```python
from build123d import *

# Parameters (mm, degrees)
F0_R     = 73.412381
F1_DEPTH = 25.4
F2_W     = 16.572997
F2_H     = 80.379516
F3_DEPTH = 25.4


with BuildPart() as f1:
    # F0 (on Top) → F1 (new body)
    with BuildSketch(Plane.XY):
        Circle(F0_R)
    extrude(amount=F1_DEPTH)

    # F2 (on face) → F3 (join)
    with BuildSketch(Plane.XY.offset(25.4)):
        with Locations((-12.828204, 0)):
            Rectangle(F2_W, F2_H)
    extrude(amount=F3_DEPTH)


solid = f1.part
```
For this review, take the finished solid that the model builds, in its own axes (mm). A direction names the side the tool comes from. Coordinates: 2 decimals unless noted, no trailing zeros. Order: outer loops, then holes, each group sorted by start corner. A loop starts at its lowest first (then second) coordinate and runs counter-clockwise, first axis right, second up. Notation, with made-up numbers: (2.25, 73.25) -> (38.25, 73.25) arc R21 ccw to (38.25, 85.25) -> close; hole circle Ø4 at (2.25, 84.25). An arc over 180 degrees is marked (long way). Answer as CSV lines item,"result".
Q1. Wall thickness on line 1 along Z through (x, y) = (4, -14); line 2 along Y through (x, z) = (-18, 40); line 3 along X through (y, z) = (11.5, 32.5): over which ranges is each line inside the solid? List them lowest first. Write a range as [from, to].
Model answer:
line 1,"z = [0, 25.4]"
line 2,"y = [-40.19, 40.19]"
line 3,"x = [-21.11, -4.54]"
Q2. We need section C-C (x = 0). State the section outline as (y, z) points, plus the area to 3 significant figures.
Model answer:
outline,"(-73.41, 0) -> (73.41, 0) -> (73.41, 25.4) -> (-73.41, 25.4) -> close"
area,"3,730 mm2"
Q3. Clearance check with flat-ended pins moving along their axes: pin 1 Ø1 at (x, z) = (-36.5, 15.5) entering from +Y; pin 2 Ø6 at (y, z) = (43, 37) entering from +X; pin 3 Ø1.5 at (x, z) = (12, 21.5) entering from +Y; pin 4 Ø6 at (x, y) = (-27.5, 47) entering from -Z. State where each tip first meets the part, or that it passes through.
Model answer:
pin 1,"stops at y = 63.98"
pin 2,"stops at x = -4.54"
pin 3,"stops at y = 72.55"
pin 4,"stops at z = 0"
Q4. For faces 1 (the face through (-13, 1, 50.8)), 2 (the face through (-21.115, -1, 38)), 3 (the face through (-4.542, -1, 38)), list the 3-axis set-ups (+Z, -Z, +X, -X, +Y, -Y) from which the entire face can be reached by the end or side of a thin tool; tool diameter is ignored.
Model answer:
face 1,"+Z, +X, -X, +Y, -Y"
face 2,"+Z, -X, +Y, -Y"
face 3,"+Z, +X, +Y, -Y"
Q5. We need section D-D (y = 34.5). State the section outline as (x, z) points, plus the area to 3 significant figures.
Model answer:
outline,"(-64.8, 0) -> (64.8, 0) -> (64.8, 25.4) -> (-4.54, 25.4) -> (-4.54, 50.8) -> (-21.11, 50.8) -> (-21.11, 25.4) -> (-64.8, 25.4) -> close"
area,"3,710 mm2"
Q6. We need section A-A (y = 0). State the section outline as (x, z) points.
Model answer:
outline,"(-73.41, 0) -> (73.41, 0) -> (73.41, 25.4) -> (-4.54, 25.4) -> (-4.54, 50.8) -> (-21.11, 50.8) -> (-21.11, 25.4) -> (-73.41, 25.4) -> close"
Q7. We need section B-B (z = 14). State the section outline as (x, y) points.
Model answer:
outline,"circle Ø146.82 at (0, 0)"
Q8. Draft analysis for pull direction Y (two halves, no side actions). For faces 4 (the face through (70.022, 22.051, 12.522)), 5 (the face through (-13, 40.19, 38)), 6 (the face through (-1, 1, 0)), 7 (the face through (-13, -40.19, 38)), state which applies: released by +Y, released by -Y, zero draft, split by the parting line, or undercut.
Model answer:
face 4,"split by the parting line"
face 5,"released by +Y"
face 6,"zero draft"
face 7,"released by -Y"
